```python
from build123d import *

# Parameters (mm, degrees)
SKETCH1_R           = 2.5527
BOSS_EXTRUDE1_DEPTH = 3.175


with BuildPart() as part:
    # Sketch1 → Boss-Extrude1 (new body)
    with BuildSketch(Plane(origin=(0, 0, 0), x_dir=(1, 0, 0), z_dir=(0, 1, 0))):
        Polygon((0, 0), (50.8, 0), (50.8, -76.2), (101.6, -76.2), (152.4, -76.2), (152.4, -25.4), (101.6, -25.4), (101.6, 50.8), (0, 50.8), align=None)
        with Locations((12.7, 25.4)):
            Circle(SKETCH1_R, mode=Mode.SUBTRACT)
        with Locations((38.1, 12.7)):
            Circle(SKETCH1_R, mode=Mode.SUBTRACT)
        with Locations((38.1, 38.1)):
            Circle(SKETCH1_R, mode=Mode.SUBTRACT)
        with Locations((139.7, -50.8)):
            Circle(SKETCH1_R, mode=Mode.SUBTRACT)
        with Locations((114.3, -38.1)):
            Circle(SKETCH1_R, mode=Mode.SUBTRACT)
        with Locations((114.3, -63.5)):
            Circle(SKETCH1_R, mode=Mode.SUBTRACT)
        with Locations((63.5, -6.35)):
            Circle(SKETCH1_R, mode=Mode.SUBTRACT)
        with Locations((88.9, -6.35)):
            Circle(SKETCH1_R, mode=Mode.SUBTRACT)
        with Locations((76.2, -19.05)):
            Circle(SKETCH1_R, mode=Mode.SUBTRACT)
    extrude(amount=BOSS_EXTRUDE1_DEPTH)


solid = part.part
```
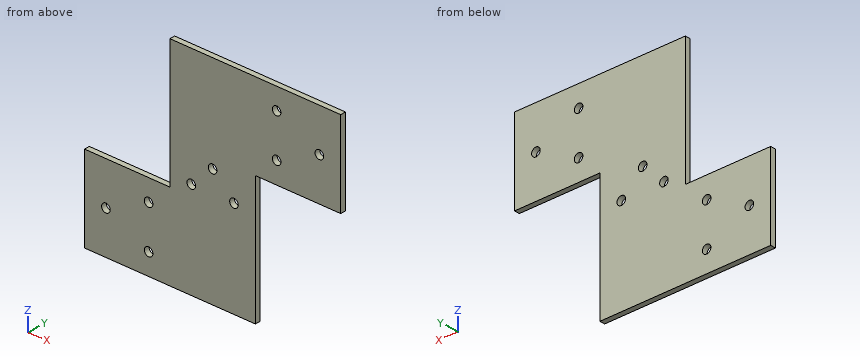
Work out the finished part from the listing and answer in its coordinate system (mm). Give positions to 0.01 mm unless a question says otherwise; leave off trailing zeros. Loops run counter-clockwise (first coordinate to the right, second up) from the corner with the lowest first, then second, coordinate; pieces in that order, holes last. Notation, with made-up numbers: (66, 56.5) -> (85, 56.5) arc R11 ccw to (85, 65.5) -> close; hole circle Ø1 at (88, -15.75). An arc over 180 degrees is marked (long way). Put each result on its own line as item: value. Start each with the question number.
Item 1: The part is cut by section D-D (y = 0.7). State how many separate pieces and enclosed holes the cut face has, then the cut area to 3 significant figures.
Item 2: Find the intervals of material crossed by L1, parallel to X at y = 1.9, z = 6.35; L2, parallel to Z at x = 114.3, y = 1.65; L3, parallel to X at y = 1.75, z = 38.1, in increasing order. Write a range as [from, to].
Item 3: This flat-tipped pin is pushed along its axis until it touches: P1, Ø1.6, axis at y = 1, z = 43, coming from the -X side. Where does it stop, or does it pass through?
Item 4: The part is cut by section A-A (z = 6.35). Give the vertices of the cut face in (x, y) (3 decimals).
Item 5: The part is cut by section B-B (x = 38.1). Give the vertices of the cut face in (y, z) (3 decimals), then the cut area to 3 significant figures.
Item 6: The part is cut by section C-C (z = 63.5). Give the vertices of the cut face in (x, y) (3 decimals), then the cut area to 3 significant figures.
Answers below:
1. separate pieces: 1
1. enclosed holes: 9
1. area: 11,400 mm2
2. L1: [50.8, 60.95], [66.05, 86.35], [91.45, 101.6]
2. L2: [25.4, 35.55], [40.65, 60.95], [66.05, 76.2]
2. L3: [50.8, 111.75], [116.85, 152.4]
3. P1: x = 50.8
4. outline: (50.8, 0) -> (60.947, 0) -> (60.947, 3.175) -> (50.8, 3.175) -> close; (66.053, 0) -> (86.347, 0) -> (86.347, 3.175) -> (66.053, 3.175) -> close; (91.453, 0) -> (101.6, 0) -> (101.6, 3.175) -> (91.453, 3.175) -> close
5. outline: (0, -50.8) -> (3.175, -50.8) -> (3.175, -40.653) -> (0, -40.653) -> close; (0, -35.547) -> (3.175, -35.547) -> (3.175, -15.253) -> (0, -15.253) -> close; (0, -10.147) -> (3.175, -10.147) -> (3.175, 0) -> (0, 0) -> close
5. area: 129 mm2
6. outline: (50.8, 0) -> (111.747, 0) -> (111.747, 3.175) -> (50.8, 3.175) -> close; (116.853, 0) -> (152.4, 0) -> (152.4, 3.175) -> (116.853, 3.175) -> close
6. area: 306 mm2
